Build history of the part. All positions in model axes, mm. Face numbers are marked on the shaded views. A direction names the side the tool comes from. Coordinates: 2 decimals unless noted, no trailing zeros. Order: outer loops, then holes, each group sorted by start corner. A loop starts at its lowest first (then second) coordinate and runs counter-clockwise, first axis right, second up. Notation, with made-up numbers: M 78.25,7.5 L 122.25,7.5 A25 cw 122.25,25.5 Z; hole C -35,60.25 d8. An arc over 180 degrees is marked long. Write item = value, one per line. Start each with the question number.
Q1. Band-saw the part on C-C on z = 21. Write the cut outline in (x, y), plus the area to 3 significant figures.
Q2. Band-saw the part on B-B on y = 6.75. Write the cut outline in (x, z), plus the area to 3 significant figures.
Q3. Band-saw the part on D-D on x = -20. Write the cut outline in (y, z), plus the area to 3 significant figures.
Q4. 3-axis set-ups, long thin cutter, end or side, ignore diameter. For the marked faces 1, 2 and 3: which of +Z, -Z, +X, -X, +Y, -Y reach the whole face in a straight line?
Q5. Band-saw the part on A-A on x = 0.5. Write the cut outline in (y, z).
Q6. Drill centre lines: probe 1 along X at (y, z) = (7, -20); probe 2 along X at (y, z) = (1.5, 22); probe 3 along Z at (x, y) = (-13, 2). Where is each one in solid material? Low to high.
Q7. Pin check, flat tips, straight feed: P1, Ø6, axis at x = 7.5, y = 6.5, coming from the -Z side; P2, Ø5, axis at x = 8.5, y = 4, coming from the -Z side. Stop position of each tip, or through.
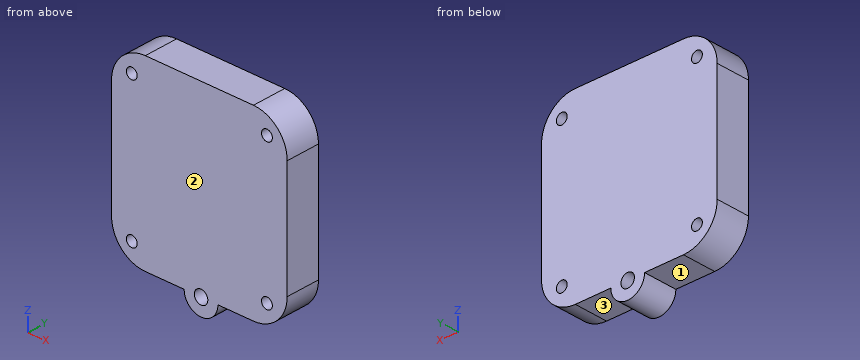
```python
from build123d import *

# Parameters (mm, degrees)
SKETCH1_R           = 1.6
SKETCH1_R_2         = 2
BOSS_EXTRUDE1_DEPTH = 10
FILLET1_R           = 10
FILLET2_R           = 10
FILLET3_R           = 10
FILLET4_R           = 10


with BuildPart() as part:
    # Sketch1 → Boss-Extrude1 (new body)
    with BuildSketch(Plane(origin=(0, 0, 0), x_dir=(1, 0, 0), z_dir=(0, 1, 0))):
        with BuildLine():
            Line((-4.5, 27), (-26, 27))
            Line((-26, 27), (-26, -27))
            Line((-26, -27), (26, -27))
            Line((26, -27), (26, 27))
            Line((26, 27), (5.5, 27))
            ThreePointArc((5.5, 27), (0.5, 32), (-4.5, 27))
        make_face()
        with Locations(Location((-20, 21, 0), (0, 0, 270))):  # turned: the seam where the file's is
            Circle(SKETCH1_R, mode=Mode.SUBTRACT)
        with Locations(Location((20, 21, 0), (0, 0, 270))):  # turned: the seam where the file's is
            Circle(SKETCH1_R, mode=Mode.SUBTRACT)
        with Locations(Location((20, -21, 0), (0, 0, 270))):  # turned: the seam where the file's is
            Circle(SKETCH1_R, mode=Mode.SUBTRACT)
        with Locations(Location((-20, -21, 0), (0, 0, 270))):  # turned: the seam where the file's is
            Circle(SKETCH1_R, mode=Mode.SUBTRACT)
        with Locations(Location((0.5, 27, 0), (0, 0, 270))):  # turned: the seam where the file's is
            Circle(SKETCH1_R_2, mode=Mode.SUBTRACT)
    extrude(amount=BOSS_EXTRUDE1_DEPTH)

    # Fillet1
    fillet1_edges = [part.edges().sort_by_distance(p)[0] for p in [
        (-26, 5, -27),
    ]]
    fillet(fillet1_edges, radius=FILLET1_R)

    # Fillet2
    fillet2_edges = [part.edges().sort_by_distance(p)[0] for p in [
        (26, 5, -27),
    ]]
    fillet(fillet2_edges, radius=FILLET2_R)

    # Fillet3
    fillet3_edges = [part.edges().sort_by_distance(p)[0] for p in [
        (-26, 5, 27),
    ]]
    fillet(fillet3_edges, radius=FILLET3_R)

    # Fillet4
    fillet4_edges = [part.edges().sort_by_distance(p)[0] for p in [
        (26, 5, 27),
    ]]
    fillet(fillet4_edges, radius=FILLET4_R)


solid = part.part
```
Recorded:
q1.outline = M -25.17,0 L -21.6,0 L -21.6,10 L -25.17,10 Z; M -18.4,0 L 18.4,0 L 18.4,10 L -18.4,10 Z; M 21.6,0 L 25.17,0 L 25.17,10 L 21.6,10 Z
q1.area = 439 mm2
q2.outline = M -26,-17 A10 ccw -16,-27 L -4.5,-27 A5 ccw 5.5,-27 L 16,-27 A10 ccw 26,-17 L 26,17 A10 ccw 16,27 L -16,27 A10 ccw -26,17 Z; hole C -20,-21 d3.2; hole C -20,21 d3.2; hole C 0.5,-27 d4; hole C 20,-21 d3.2; hole C 20,21 d3.2
q2.area = 2,720 mm2
q3.outline = M 0,-26.17 L 10,-26.17 L 10,-22.6 L 0,-22.6 Z; M 0,-19.4 L 10,-19.4 L 10,19.4 L 0,19.4 Z; M 0,22.6 L 10,22.6 L 10,26.17 L 0,26.17 Z
q3.area = 459 mm2
q4.face_1 = -Z, -X, +Y, -Y
q4.face_2 = +Z, -Z, +X, -X, -Y
q4.face_3 = -Z, +X, +Y, -Y
q5.outline = M 0,-32 L 10,-32 L 10,-29 L 0,-29 Z; M 0,-25 L 10,-25 L 10,27 L 0,27 Z
q6.probe_1 = -25.54 to -21.25, -18.75 to 18.75, 21.25 to 25.54
q6.probe_2 = -24.66 to -21.25, -18.75 to 18.75, 21.25 to 24.66
q6.probe_3 = -27 to 27
q7.P1 = -30
q7.P2 = -27
